Part print with two shaded views. Sizes in mm from the minimum x, y, z corner. Round coordinates to 2 decimals unless told otherwise and drop trailing zeros. Write each loop counter-clockwise with the first axis right and the second up, starting at its lowest first coordinate (ties: lowest second). Pieces come first, ordered by that corner, then holes. Notation, with made-up numbers: M -21,34 L 30,34 A25 cw 30,47 Z; hole C 59,61.5 d11. An arc over 180 degrees is marked long. Use one line per item in the form item = value. Start each with the question number.
Item 1: Flat gauge pins, fed straight in: pin 1 Ø6 at (x, z) = (70, 25) entering from -Y; pin 2 Ø3 at (x, y) = (50.5, 4) entering from +Z; pin 3 Ø1.6 at (x, z) = (32.5, 57) entering from +Y. Where does each tip first touch, or does it go through?
Item 2: Cut at C-C, the plane z = 27.5. Give the cut face in (x, y).
Item 3: Probe L1, parallel to Z at x = 38, y = 4.7; L2, parallel to Y at x = 19, z = 27; L3, parallel to Z at x = 45, y = 4.65. List the from-to ranges inside material, lowest first.
Item 4: Cut at A-A, the plane y = 0.95. Give the cut face in (x, z).
Item 5: Cut at B-B, the plane x = 61. Give the cut face in (y, z).
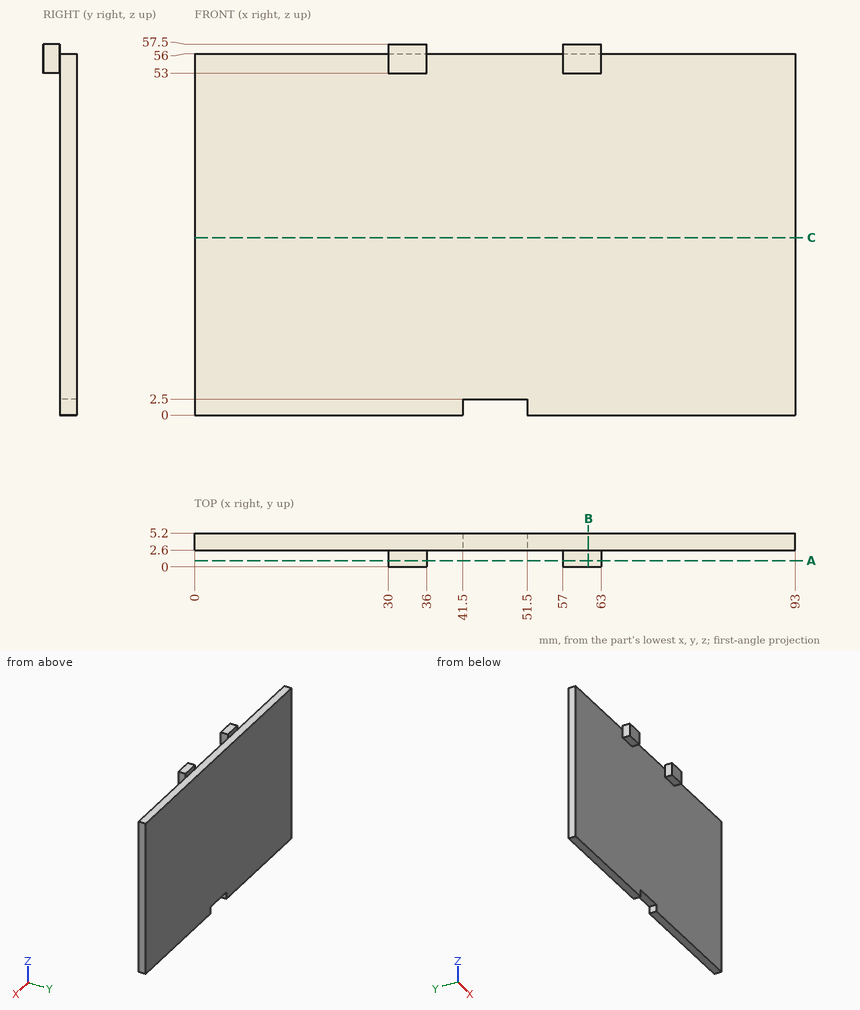
Model answer:
q1.pin_1 = 2.6
q1.pin_2 = 56
q1.pin_3 = 2.6
q2.outline = M 0,2.6 L 93,2.6 L 93,5.2 L 0,5.2 Z
q3.L1 = 0 to 56
q3.L2 = 2.6 to 5.2
q3.L3 = 2.5 to 56
q4.outline = M 30,53 L 36,53 L 36,57.5 L 30,57.5 Z; M 57,53 L 63,53 L 63,57.5 L 57,57.5 Z
q5.outline = M 0,53 L 2.6,53 L 2.6,0 L 5.2,0 L 5.2,56 L 2.6,56 L 2.6,57.5 L 0,57.5 Z
